For this review, take the finished solid that the model builds, in its own axes (mm). A direction names the side the tool comes from. Coordinates: 2 decimals unless noted, no trailing zeros. Loops run counter-clockwise (first coordinate to the right, second up) from the corner with the lowest first, then second, coordinate; pieces in that order, holes last.
1. Take a section at A-A, the plane y = 0. State the section outline as (x, z) points, then the cut area to 3 significant figures.
2. Clearance check with flat-ended pins moving along their axes: P1, Ø2, axis at y = 2, z = 1, coming from the +X side; P2, Ø2, axis at y = 1.5, z = 3.5, coming from the +X side. State where each tip first meets the part, or that it passes through.
3. To check wall thickness, follow probe 1 along Y at (x, z) = (0, 0.15); probe 2 along Y at (x, z) = (0, 0.1); probe 3 along Z at (x, y) = (-0.35, -1.8). State the ranges of each line that lie inside material, in increasing order.
4. Machinability: for faces 3 (the face through (0.715, -1.375, 2.726)), 4 (the face through (0, 0, 4.5)), which of the approach directions +Z, -Z, +X, -X, +Y, -Y give a long, thin tool a straight path to every point of the face, cutting with its end or side? Answer none if there is none.
5. Mouldability with a two-part tool opening along Y and no side actions: class faces 1 (the face through (-3, 0.1, 0.7)), 2 (the face through (1.3, -1.3, 1)) as pulls with the +Y half, pulls with the -Y half, needs draft (parallel to the pull), parting line crosses it, or undercut.
6. Take a section at D-D, the plane z = 0.9. State the section outline as (x, y) points.
7. Take a section at C-C, the plane z = 3.2. State the section outline as (x, y) points, then the cut area to 3 significant figures.
```python
from build123d import *

# Parameters (mm, degrees)
SKETCH1_R           = 3
BOSS_EXTRUDE1_DEPTH = 1
SKETCH2_R           = 1.55
BOSS_EXTRUDE2_DEPTH = 3.5
CHAMFER1_SIZE       = 0.7
CHAMFER1_SIZE2      = 0.404145188
SKETCH3_R           = 1.15
CUT_EXTRUDE1_DEPTH  = 0.2
SKETCH4_R           = 0.85
BOSS_EXTRUDE3_DEPTH = 0.2


with BuildPart() as part:
    # Sketch1 → Boss-Extrude1 (new body)
    with BuildSketch(Plane.XY):
        Circle(SKETCH1_R)
    extrude(amount=BOSS_EXTRUDE1_DEPTH)

    # Sketch2 → Boss-Extrude2 (add)
    with BuildSketch(Plane.XY.offset(1)):
        Circle(SKETCH2_R)
    extrude(amount=BOSS_EXTRUDE2_DEPTH)

    # Chamfer1
    chamfer1_edges = [part.edges().sort_by_distance(p)[0] for p in [
        (-3, 0, 0),
    ]]
    chamfer1_side = [part.faces().sort_by_distance(p)[0] for p in [
        (0, 0, 0),
    ]]
    chamfer(chamfer1_edges, length=CHAMFER1_SIZE, length2=CHAMFER1_SIZE2, reference=chamfer1_side[0])

    # Sketch3 → Cut-Extrude1 (cut)
    with BuildSketch(Plane(origin=(0, 0, 0), x_dir=(-1, 0, 0), z_dir=(0, 0, -1))):
        Circle(SKETCH3_R)
    extrude(amount=-CUT_EXTRUDE1_DEPTH, mode=Mode.SUBTRACT)

    # Sketch4 → Boss-Extrude3 (add)
    with BuildSketch(Plane(origin=(0, 0, 0.2), x_dir=(-1, 0, 0), z_dir=(0, 0, -1))):
        Circle(SKETCH4_R)
    extrude(amount=BOSS_EXTRUDE3_DEPTH)


solid = part.part
```
Results list:
1. outline: (-3, 0.4) - (-2.3, 0) - (-1.15, 0) - (-1.15, 0.2) - (-0.85, 0.2) - (-0.85, 0) - (0.85, 0) - (0.85, 0.2) - (1.15, 0.2) - (1.15, 0) - (2.3, 0) - (3, 0.4) - (3, 1) - (1.55, 1) - (1.55, 4.5) - (-1.55, 4.5) - (-1.55, 1) - (-3, 1) - close
1. area: 16.4 mm2
2. P1: stops at x = 2.83
2. P2: stops at x = 1.47
3. probe 1: y = -2.56 to -1.15, -0.85 to 0.85, 1.15 to 2.56
3. probe 2: y = -2.47 to -1.15, -0.85 to 0.85, 1.15 to 2.47
3. probe 3: z = 0 to 1
4. face 3: +Z
4. face 4: +Z, +X, -X, +Y, -Y
5. face 1: parting line crosses it
5. face 2: needs draft
6. outline: circle Ø6 at (0, 0)
7. outline: circle Ø3.1 at (0, 0)
7. area: 7.55 mm2
